from build123d import *

# Parameters (mm, degrees)
ESBO_O1_W                 = 181.6
ESBO_O1_H                 = 103.1
RESSALTO_EXTRUS_O1_DEPTH  = 10
ESBO_O2_W                 = 178.6
ESBO_O2_H                 = 100.1
CORTE_EXTRUS_O1_DEPTH     = 7
ESBO_O4_W                 = 4.8
ESBO_O4_H                 = 9.8
RESSALTO_EXTRUS_O2_DEPTH  = 2
ESPELHAR2_COPY_1_SKETCH_W = 4.8
ESPELHAR2_COPY_1_SKETCH_H = 9.8
ESPELHAR2_COPY_1_DEPTH    = 2
ESBO_O5_W                 = 10
ESBO_O5_H                 = 181.6
CORTE_EXTRUS_O2_DEPTH     = 3
FILETE3_R                 = 1
FILETE6_R                 = 1
FILETE7_R                 = 1
FILETE8_R                 = 1
ESBO_O6_R                 = 13.2
CORTE_EXTRUS_O3_DEPTH     = 10


with BuildPart() as part:
    # Esboço1 → Ressalto-extrusão1 (new body)
    with BuildSketch(Plane.YZ):
        Rectangle(ESBO_O1_W, ESBO_O1_H)
    extrude(amount=RESSALTO_EXTRUS_O1_DEPTH)

    # Esboço2 → Corte-extrusão1 (cut)
    with BuildSketch(Plane.YZ.offset(10)):
        Rectangle(ESBO_O2_W, ESBO_O2_H)
    extrude(amount=-CORTE_EXTRUS_O1_DEPTH, mode=Mode.SUBTRACT)

    # Esboço4 → Ressalto-extrusão2 (add)
    with BuildSketch(Plane(origin=(0, -89.3, 0), x_dir=(-1, 0, 0), z_dir=(0, 1, 0))):
        with Locations((-7.6, 35.1)):
            Rectangle(ESBO_O4_W, ESBO_O4_H)
    ressalto_extrus_o2 = extrude(amount=RESSALTO_EXTRUS_O2_DEPTH)

    # Espelhar1: Ressalto-extrusão2 across plane
    add(ressalto_extrus_o2.mirror(Plane.XY))

    # Espelhar2: Ressalto-extrusão2 across plane
    add(ressalto_extrus_o2.mirror(Plane.ZX))

    # Espelhar2 copy 1 sketch → Espelhar2 copy 1 (add)
    with BuildSketch(Plane(origin=(0, 89.3, 0), x_dir=(-1, 0, 0), z_dir=(0, -1, 0))):
        with Locations((-7.6, 35.1)):
            Rectangle(ESPELHAR2_COPY_1_SKETCH_W, ESPELHAR2_COPY_1_SKETCH_H)
    extrude(amount=ESPELHAR2_COPY_1_DEPTH)

    # Esboço5 → Corte-extrusão2 (cut)
    with BuildSketch(Plane(origin=(0, 0, -51.55), x_dir=(1, 0, 0), z_dir=(0, 0, -1))):
        with Locations((5, 0)):
            Rectangle(ESBO_O5_W, ESBO_O5_H)
    extrude(amount=-CORTE_EXTRUS_O2_DEPTH, mode=Mode.SUBTRACT)

    # Filete3
    filete3_edges = [part.edges().sort_by_distance(p)[0] for p in [
        (10, 0, 51.55),
        (10, -90.8, 1.5),
        (0, 0, 51.55),
        (0, -90.8, 1.5),
        (5, 90.8, 51.55),
        (0, 90.8, 1.5),
        (10, 90.8, 1.5),
        (0, 0, -48.55),
        (5, -90.8, -48.55),
        (5, 90.8, -48.55),
    ]]
    fillet(filete3_edges, radius=FILETE3_R)

    # Filete6
    filete6_edges = [part.edges().sort_by_distance(p)[0] for p in [
        (5.2, -87.3, 35.1),
        (7.6, -87.3, 40),
        (10, -87.3, 35.1),
        (7.6, -87.3, 30.2),
    ]]
    fillet(filete6_edges, radius=FILETE6_R)

    # Filete7
    filete7_edges = [part.edges().sort_by_distance(p)[0] for p in [
        (10, -87.3, -35.1),
        (7.6, -87.3, -30.2),
        (7.6, -87.3, -40),
        (5.2, -87.3, -35.1),
    ]]
    fillet(filete7_edges, radius=FILETE7_R)

    # Filete8
    filete8_edges = [part.edges().sort_by_distance(p)[0] for p in [
        (5.2, 87.3, -35.1),
        (7.6, 87.3, -40),
        (10, 87.3, -35.1),
        (7.6, 87.3, -30.2),
        (10, 87.3, 35.1),
        (7.6, 87.3, 30.2),
        (7.6, 87.3, 40),
        (5.2, 87.3, 35.1),
    ]]
    fillet(filete8_edges, radius=FILETE8_R)

    # Esboço6 → Corte-extrusão3 (cut)
    with BuildSketch(Plane(origin=(0, 0, 0), x_dir=(0, -1, 0), z_dir=(-1, 0, 0))):
        with Locations(Location((-71.25, -22.55, 0), (0, 0, 90))):
            Circle(ESBO_O6_R)
    corte_extrus_o3 = extrude(amount=-CORTE_EXTRUS_O3_DEPTH, mode=Mode.SUBTRACT)

    # Espelhar3: Corte-extrusão3 across plane
    add(corte_extrus_o3.mirror(Plane.ZX), mode=Mode.SUBTRACT)


solid = part.part
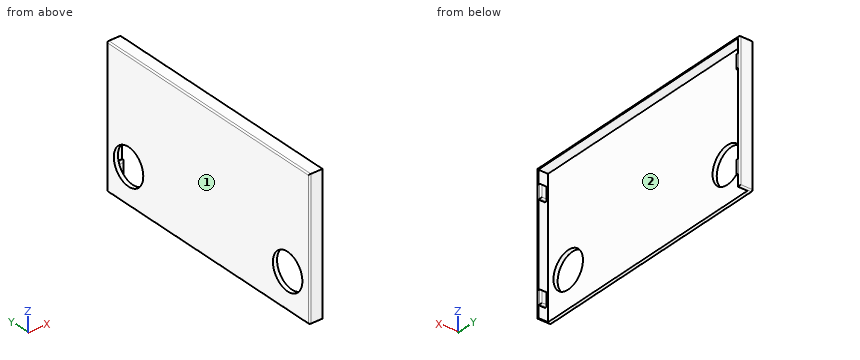
CAD build for the part. Positions are in the model's coordinates, mm. Face numbers are marked on the shaded views. Coordinates: 2 decimals unless noted, no trailing zeros. Write each loop counter-clockwise with the first axis right and the second up, starting at its lowest first coordinate (ties: lowest second). Pieces come first, ordered by that corner, then holes. Notation, with made-up numbers: M 14.25,-11.75 L 52.25,-11.75 A25 ccw 52.25,9.25 Z; hole C -35,-7.75 d3. An arc over 180 degrees is marked long. Answer as a JSON object with one key per item and string values. Group by question number.
1) Saw through at B-B (z = -22.55). Write the cut outline in (x, y).
2) Saw through at D-D (z = 14.5). Write the cut outline in (x, y).
3) Mould opens along Y. For the marked faces 1 and 2 say: +Y half, -Y half, draft (parallel to the pull), parting line (faces both ways), or undercut.
4) Wall check: line 1 (Y direction, x = 0.8, z = -22.55); line 2 (Y direction, x = 5, z = -4.5); line 3 (Z direction, x = 1.4, y = -71.25). Give the ranges that are in metal, low to high. Write a range as from..to.
5) Saw through at A-A (y = 71.25). Write the cut outline in (x, z), plus the area to 3 significant figures.
6) Saw through at C-C (y = 49). Write the cut outline in (x, z).
7) Pin check, flat tips, straight feed: pin 1 Ø16 at (y, z) = (71.25, -22.55) entering from +X; pin 2 Ø6 at (y, z) = (35, -1) entering from +X; pin 3 Ø2 at (x, y) = (7.5, 31.5) entering from -Z; pin 4 Ø1.1 at (x, y) = (8, -88.5) entering from -Z. Stop position of each tip, or through.
Values follow:
{
 "1": {"outline": "M 0,-89.8 A1 ccw 1,-90.8 L 9,-90.8 A1 ccw 10,-89.8 L 10,-89.3 L 3,-89.3 L 3,-84.45 L 0,-84.45 Z; M 0,-58.05 L 3,-58.05 L 3,58.05 L 0,58.05 Z; M 0,84.45 L 3,84.45 L 3,89.3 L 10,89.3 L 10,89.8 A1 ccw 9,90.8 L 1,90.8 A1 ccw 0,89.8 Z"},
 "2": {"outline": "M 0,-89.8 A1 ccw 1,-90.8 L 9,-90.8 A1 ccw 10,-89.8 L 10,-89.3 L 3,-89.3 L 3,89.3 L 10,89.3 L 10,89.8 A1 ccw 9,90.8 L 1,90.8 A1 ccw 0,89.8 Z"},
 "3": {"face 1": "draft", "face 2": "undercut"},
 "4": {"line 1": "y = -90.78..-84.45, -58.05..58.05, 84.45..90.78", "line 2": "y = -90.8..-89.3, 89.3..90.8", "line 3": "z = -48.55..-35.75, -9.35..51.55"},
 "5": {"outline": "M 0,-47.55 A1 ccw 1,-48.55 L 3,-48.55 L 3,-35.75 L 0,-35.75 Z; M 0,-9.35 L 3,-9.35 L 3,50.05 L 10,50.05 L 10,50.55 A1 ccw 9,51.55 L 1,51.55 A1 ccw 0,50.55 Z", "area": "231 mm2"},
 "6": {"outline": "M 0,-47.55 A1 ccw 1,-48.55 L 3,-48.55 L 3,50.05 L 10,50.05 L 10,50.55 A1 ccw 9,51.55 L 1,51.55 A1 ccw 0,50.55 Z"},
 "7": {"pin 1": "passes through", "pin 2": "stops at x = 3", "pin 3": "stops at z = 50.05", "pin 4": "stops at z = -40"}
}
